```python
from build123d import *

# Parameters (mm, degrees)
SKETCH2_R           = 3.175
BOSS_EXTRUDE1_DEPTH = 6.35
SKETCH3_W           = 3.175
SKETCH3_H           = 6.604
CUT_EXTRUDE1_DEPTH  = 551.59524986


with BuildPart() as part:
    # Sketch2 → Boss-Extrude1 (new body)
    with BuildSketch(Plane(origin=(0, 0, 0), x_dir=(0, 0, -1), z_dir=(1, 0, 0))):
        with BuildLine():
            Line((12.003150763, 442.097734975), (138.953150763, 442.097734975))
            Line((138.953150763, 442.097734975), (138.953150763, 452.097734975))
            ThreePointArc((138.953150763, 452.097734975), (148.953150763, 462.097734975), (158.953150763, 452.097734975))
            Line((158.953150763, 452.097734975), (158.953150763, 442.097734975))
            Line((158.953150763, 442.097734975), (298.603150763, 442.097734975))
            Line((298.603150763, 442.097734975), (298.603150763, 389.397734975))
            Line((298.603150763, 389.397734975), (304.953150763, 389.397734975))
            Line((304.953150763, 389.397734975), (304.953150763, 409.397734975))
            Line((304.953150763, 409.397734975), (311.303150763, 409.397734975))
            Line((311.303150763, 409.397734975), (311.303150763, 375.747734975))
            Line((311.303150763, 375.747734975), (304.953150763, 369.397734975))
            Line((304.953150763, 369.397734975), (298.603150763, 369.397734975))
            Line((298.603150763, 369.397734975), (298.603150763, 234.397734975))
            Line((298.603150763, 234.397734975), (304.953150763, 234.397734975))
            Line((304.953150763, 234.397734975), (304.953150763, 254.397734975))
            Line((304.953150763, 254.397734975), (311.303150763, 254.397734975))
            Line((311.303150763, 254.397734975), (311.303150763, 220.747734975))
            Line((311.303150763, 220.747734975), (304.953150763, 214.397734975))
            Line((304.953150763, 214.397734975), (298.603150763, 214.397734975))
            Line((298.603150763, 214.397734975), (298.603150763, 79.397734975))
            Line((298.603150763, 79.397734975), (304.953150763, 79.397734975))
            Line((304.953150763, 79.397734975), (304.953150763, 99.397734975))
            Line((304.953150763, 99.397734975), (311.303150763, 99.397734975))
            Line((311.303150763, 99.397734975), (311.303150763, 65.747734975))
            Line((311.303150763, 65.747734975), (304.953150763, 59.397734975))
            Line((304.953150763, 59.397734975), (298.603150763, 59.397734975))
            Line((298.603150763, 59.397734975), (298.603150763, -15.602265025))
            Line((298.603150763, -15.602265025), (223.103150763, -15.602265025))
            Line((223.103150763, -15.602265025), (223.103150763, -21.952265025))
            Line((223.103150763, -21.952265025), (243.103150763, -21.952265025))
            Line((243.103150763, -21.952265025), (243.103150763, -28.302265025))
            Line((243.103150763, -28.302265025), (209.453150763, -28.302265025))
            Line((209.453150763, -28.302265025), (203.103150763, -21.952265025))
            Line((203.103150763, -21.952265025), (203.103150763, -15.602265025))
            Line((203.103150763, -15.602265025), (107.603150763, -15.602265025))
            Line((107.603150763, -15.602265025), (107.603150763, -21.952265025))
            Line((107.603150763, -21.952265025), (127.603150763, -21.952265025))
            Line((127.603150763, -21.952265025), (127.603150763, -28.302265025))
            Line((127.603150763, -28.302265025), (93.953150763, -28.302265025))
            Line((93.953150763, -28.302265025), (87.603150763, -21.952265025))
            Line((87.603150763, -21.952265025), (87.603150763, -15.602265025))
            Line((87.603150763, -15.602265025), (12.003150763, -15.602265025))
            Line((12.003150763, -15.602265025), (12.003150763, 59.397734975))
            Line((12.003150763, 59.397734975), (5.653150763, 59.397734975))
            Line((5.653150763, 59.397734975), (-0.696849237, 65.747734975))
            Line((-0.696849237, 65.747734975), (-0.696849237, 99.397734975))
            Line((-0.696849237, 99.397734975), (5.653150763, 99.397734975))
            Line((5.653150763, 99.397734975), (5.653150763, 79.397734975))
            Line((5.653150763, 79.397734975), (12.003150763, 79.397734975))
            Line((12.003150763, 79.397734975), (12.003150763, 214.366115656))
            Line((12.003150763, 214.366115656), (12.003150763, 214.397734975))
            Line((12.003150763, 214.397734975), (5.653150763, 214.397734975))
            Line((5.653150763, 214.397734975), (-0.696849237, 220.747734975))
            Line((-0.696849237, 220.747734975), (-0.696849237, 254.397734975))
            Line((-0.696849237, 254.397734975), (5.653150763, 254.397734975))
            Line((5.653150763, 254.397734975), (5.653150763, 234.397734975))
            Line((5.653150763, 234.397734975), (12.003150763, 234.397734975))
            Line((12.003150763, 234.397734975), (12.003150763, 369.397734975))
            Line((12.003150763, 369.397734975), (5.313181696, 369.397734975))
            Line((5.313181696, 369.397734975), (-0.696849237, 375.407765908))
            Line((-0.696849237, 375.407765908), (-0.696849237, 409.397734975))
            Line((-0.696849237, 409.397734975), (5.653150763, 409.397734975))
            Line((5.653150763, 409.397734975), (5.653150763, 389.397734975))
            Line((5.653150763, 389.397734975), (12.003150763, 389.397734975))
            Line((12.003150763, 389.397734975), (12.003150763, 442.097734975))
        make_face()
        with Locations((148.953150763, 452.097734975)):
            Circle(SKETCH2_R, mode=Mode.SUBTRACT)
    extrude(amount=BOSS_EXTRUDE1_DEPTH)

    # Sketch3 → Cut-Extrude1 (cut, through all)
    with BuildSketch(Plane.XY.offset(-12.003150763)):
        with Locations((1.5875, 432.699734975)):
            Rectangle(SKETCH3_W, SKETCH3_H)
    extrude(amount=-CUT_EXTRUDE1_DEPTH, mode=Mode.SUBTRACT)


solid = part.part
```
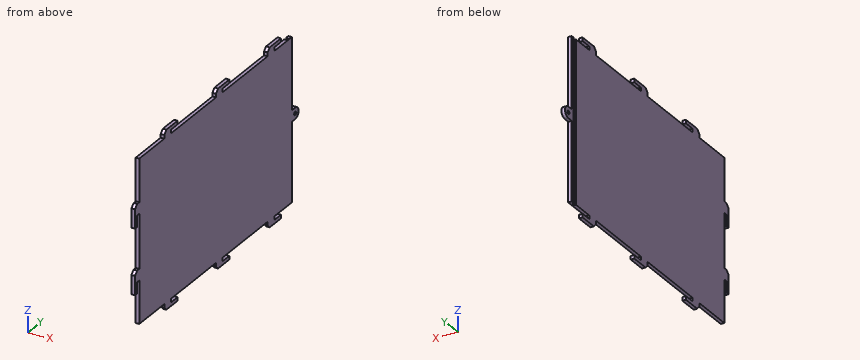
Part model, mm, in its own coordinate system. Coordinates: 2 decimals unless noted, no trailing zeros. Loops run counter-clockwise (first coordinate to the right, second up) from the corner with the lowest first, then second, coordinate; pieces in that order, holes last. Notation, with made-up numbers: (10, -35.5) - (15, -35.5) arc R16 cw to (15, -22.5) - close; hole circle Ø3 at (-21.5, 72.25). An arc over 180 degrees is marked (long way). Write item = value, one per line. Start each with the question number.
Item 1: Wall check: L1, parallel to Z at x = 3.75, y = 249; L2, parallel to Y at x = 5.5, z = -115.5; L3, parallel to Y at x = 2.5, z = -43.5. Give the ranges that are in metal, low to high. Write a range as from..to.
Item 2: Flat gauge pins, fed straight in: pin 1 Ø1.9 at (x, z) = (2, -7.5) entering from +Y; pin 2 Ø1.9 at (x, y) = (2.5, 425.5) entering from +Z; pin 3 Ø8.5 at (y, z) = (452.1, -148.95) entering from +X; pin 4 Ø3 at (x, y) = (3.5, -20) entering from -Z. Where does each tip first touch, or does it go through?
Item 3: Cut at A-A, the plane y = 395.5. Give the cut face in (x, z).
Item 4: Cut at C-C, the plane z = -75.5. Give the cut face in (x, y) (3 decimals).
Item 5: Cut at B-B, the plane x = 1. State how many separate pieces and enclosed holes the cut face has, and give its area (3 significant figures).
The answers:
q1.L1 = -311.3..-304.95, -298.6..-12, -5.65..0.7
q1.L2 = -28.3..-21.95, -15.6..442.1
q1.L3 = -15.6..429.4, 436..442.1
q2.pin_1 = 389.4
q2.pin_2 = -12
q2.pin_3 = 6.35
q2.pin_4 = -223.1
q3.outline = (0, -311.3) - (6.35, -311.3) - (6.35, -304.95) - (0, -304.95) - close; (0, -298.6) - (6.35, -298.6) - (6.35, -12) - (0, -12) - close; (0, -5.65) - (6.35, -5.65) - (6.35, 0.7) - (0, 0.7) - close
q4.outline = (0, -15.602) - (6.35, -15.602) - (6.35, 442.098) - (0, 442.098) - (0, 436.002) - (3.175, 436.002) - (3.175, 429.398) - (0, 429.398) - close
q5.separate_pieces = 2
q5.enclosed_holes = 1
q5.area = 132,000 mm2
